For this review, take the finished solid that the model builds, in its own axes (mm). A direction names the side the tool comes from. Round coordinates to 2 decimals unless told otherwise and drop trailing zeros. Order: outer loops, then holes, each group sorted by start corner. A loop starts at its lowest first (then second) coordinate and runs counter-clockwise, first axis right, second up.
```python
from build123d import *

# Parameters (mm, degrees)
SKETCH1_W                 = 32.5
SKETCH1_H                 = 52
BOSS_EXTRUDE1_DEPTH       = 5
F_2_56_TAPPED_HOLE1_D     = 1.778
F_2_56_TAPPED_HOLE1_DEPTH = 7.46583491
F_2_56_TAPPED_HOLE1_TIP   = 0.53416509
F_2_56_TAPPED_HOLE2_D     = 1.778
F_2_56_TAPPED_HOLE2_DEPTH = 7.46583491
F_2_56_TAPPED_HOLE2_TIP   = 0.53416509
CUT_EXTRUDE2_DEPTH        = 2.5
SKETCH10_R                = 3.5
CUT_EXTRUDE3_DEPTH        = 2.5


with BuildPart() as part:
    # Sketch1 → Boss-Extrude1 (new body)
    with BuildSketch(Plane(origin=(0, 0, 0), x_dir=(1, 0, 0), z_dir=(0, 1, 0))):
        with Locations((16.25, 26)):
            Rectangle(SKETCH1_W, SKETCH1_H)
    extrude(amount=BOSS_EXTRUDE1_DEPTH)

    # #2-56 Tapped Hole1
    with Locations(Plane.ZY):
        with Locations((-39, 2.5), (-13, 2.5)):
            Hole(F_2_56_TAPPED_HOLE1_D / 2, depth=F_2_56_TAPPED_HOLE1_DEPTH)
            with Locations((0, 0, -(F_2_56_TAPPED_HOLE1_DEPTH + F_2_56_TAPPED_HOLE1_TIP / 2))):  # 118° drill point
                Cone(0, F_2_56_TAPPED_HOLE1_D / 2, F_2_56_TAPPED_HOLE1_TIP, mode=Mode.SUBTRACT)

    # #2-56 Tapped Hole2
    with Locations(Plane(origin=(32.5, 0, 0), x_dir=(0, 0, -1), z_dir=(1, 0, 0))):
        with Locations((13, 2.5), (39, 2.5)):
            Hole(F_2_56_TAPPED_HOLE2_D / 2, depth=F_2_56_TAPPED_HOLE2_DEPTH)
            with Locations((0, 0, -(F_2_56_TAPPED_HOLE2_DEPTH + F_2_56_TAPPED_HOLE2_TIP / 2))):  # 118° drill point
                Cone(0, F_2_56_TAPPED_HOLE2_D / 2, F_2_56_TAPPED_HOLE2_TIP, mode=Mode.SUBTRACT)

    # Sketch11 → Cut-Extrude2 (cut)
    with BuildSketch(Plane(origin=(0, 0, 0), x_dir=(-1, 0, 0), z_dir=(0, -1, 0))):
        Polygon((-21.05, 6.57), (-21.05, 10.57), (-11.45, 10.57), (-11.45, 2.57), (-21.05, 2.57), align=None)
    extrude(amount=-CUT_EXTRUDE2_DEPTH, mode=Mode.SUBTRACT)

    # Sketch10 → Cut-Extrude3 (cut)
    with BuildSketch(Plane(origin=(0, 5, 0), x_dir=(1, 0, 0), z_dir=(0, 1, 0))):
        with Locations((16.25, 6.57)):
            Circle(SKETCH10_R)
    extrude(amount=-CUT_EXTRUDE3_DEPTH, mode=Mode.SUBTRACT)


solid = part.part
```
Q1. Take a section at A-A, the plane z = -6.57. State the section outline as (x, y) points, plus the area to 3 significant figures.
Q2. Wall thickness on line 1 (Z direction, x = 26.5, y = 2.5); line 2 (X direction, y = 0.85, z = -5); line 3 (Z direction, x = 27, y = 2.1): over which ranges is each line inside the solid? List them lowest first.
Q3. Take a section at D-D, the plane x = 30.5. State the section outline as (y, z) points.
Q4. Tool access review of faces 1 (the face through (0, 2, -26)), 2 (the face through (3.79, 2.54, -12.11)), 3 (the face through (28.71, 2.54, -13.89)), 4 (the face through (16, 1, -10.57)): name each direction out of +Z, -Z, +X, -X, +Y, -Y from which nothing blocks a thin tool from reaching the whole face with its end or side.
Q5. Clearance check with flat-ended pins moving along their axes: pin 1 (1.6 mm diameter, centred on y = 2.5, z = -39, fed in from +X); pin 2 (4 mm diameter, centred on x = 17, z = -8, fed in from -Y). State where each tip first meets the part, or that it passes through.
Q6. Take a section at B-B, the plane x = 16.25. State the section outline as (y, z) points.
Q7. Take a section at C-C, the plane y = 4.4. State the section outline as (x, z) points.
Q8. Mouldability with a two-part tool opening along Z and no side actions: class faces 5 (the face through (16, 5, -26)), 6 (the face through (24.59, 2.44, -13.14)), 7 (the face through (16, 2, 0)) as +Z half, -Z half, draft (parallel to the pull), parting line (faces both ways), or undercut.
Working result:
1. outline: (0, 0) - (11.45, 0) - (11.45, 2.5) - (12.75, 2.5) - (12.75, 5) - (0, 5) - close; (19.75, 2.5) - (21.05, 2.5) - (21.05, 0) - (32.5, 0) - (32.5, 5) - (19.75, 5) - close
1. area: 121 mm2
2. line 1: z = -52 to -39.89, -38.11 to -13.89, -12.11 to 0
2. line 2: x = 0 to 11.45, 21.05 to 32.5
2. line 3: z = -52 to -39.79, -38.21 to -13.79, -12.21 to 0
3. outline: (0, -52) - (5, -52) - (5, 0) - (0, 0) - close; hole circle Ø1.78 at (2.5, -39); hole circle Ø1.78 at (2.5, -13)
4. face 1: +Z, -Z, -X, +Y, -Y
4. face 2: -X
4. face 3: +X
4. face 4: -Y
5. pin 1: stops at x = 24.98
5. pin 2: stops at y = 2.5
6. outline: (0, -52) - (5, -52) - (5, -10.07) - (2.5, -10.07) - (2.5, -10.57) - (0, -10.57) - close; (0, -2.57) - (2.5, -2.57) - (2.5, -3.07) - (5, -3.07) - (5, 0) - (0, 0) - close
7. outline: (0, -52) - (32.5, -52) - (32.5, 0) - (0, 0) - close; hole circle Ø7 at (16.25, -6.57)
8. face 5: draft
8. face 6: undercut
8. face 7: +Z half
